from build123d import *

# Parameters (mm, degrees)
SKETCH1_R           = 250
SKETCH1_R_2         = 162.5
BOSS_EXTRUDE1_DEPTH = 19
CUT_EXTRUDE1_START  = -6
SKETCH2_R           = 250
SKETCH2_R_2         = 236
CUT_EXTRUDE1_DEPTH  = 6
SKETCH3_R           = 5
CUT_EXTRUDE2_DEPTH  = 355.063553617


with BuildPart() as part:
    # Sketch1 → Boss-Extrude1 (new body)
    with BuildSketch(Plane(origin=(0, 0, 0), x_dir=(1, 0, 0), z_dir=(0, 1, 0))):
        with Locations(Location((0, 0, 0), (0, 0, 270))):
            Circle(SKETCH1_R)
        with Locations(Location((0, 0, 0), (0, 0, 270))):
            Circle(SKETCH1_R_2, mode=Mode.SUBTRACT)
    extrude(amount=BOSS_EXTRUDE1_DEPTH)

    # Sketch2 → Cut-Extrude1 (cut)
    with BuildSketch(Plane(origin=(0, 19, 0), x_dir=(1, 0, 0), z_dir=(0, 1, 0)).offset(CUT_EXTRUDE1_START)):
        with Locations(Location((0, 0, 0), (0, 0, 270))):
            Circle(SKETCH2_R)
        with Locations(Location((0, 0, 0), (0, 0, 270))):
            Circle(SKETCH2_R_2, mode=Mode.SUBTRACT)
    extrude(amount=CUT_EXTRUDE1_DEPTH, mode=Mode.SUBTRACT)

    # Sketch3 → Cut-Extrude2 (cut, through all)
    with BuildSketch(Plane(origin=(0, 19, 0), x_dir=(1, 0, 0), z_dir=(0, 1, 0))):
        with Locations(Location((111.25, 192.690652342, 0), (0, 0, 270))):
            Circle(SKETCH3_R)
        with Locations(Location((111.25, -192.690652342, 0), (0, 0, 90))):
            Circle(SKETCH3_R)
        with Locations(Location((-111.25, -192.690652342, 0), (0, 0, 270))):
            Circle(SKETCH3_R)
        with Locations(Location((222.5, 0, 0), (0, 0, 270))):
            Circle(SKETCH3_R)
        with Locations(Location((-111.25, 192.690652342, 0), (0, 0, 90))):
            Circle(SKETCH3_R)
        with Locations(Location((-222.5, 0, 0), (0, 0, 90))):
            Circle(SKETCH3_R)
    extrude(amount=-CUT_EXTRUDE2_DEPTH, mode=Mode.SUBTRACT)


solid = part.part
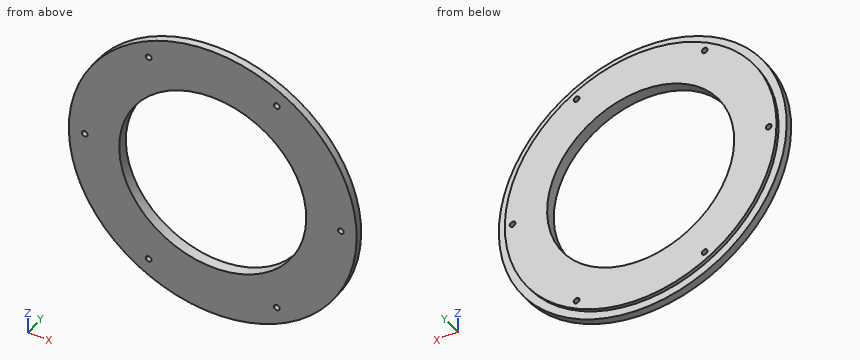
Check sheet for the modelled part. Datum: model origin and axes. Units: mm. Give positions to 0.01 mm unless a question says otherwise; leave off trailing zeros. Loops run counter-clockwise (first coordinate to the right, second up) from the corner with the lowest first, then second, coordinate; pieces in that order, holes last. Notation, with made-up numbers: M -6.75,40 L 5.25,40 A33 ccw 5.25,73 Z; hole C 27.5,22 d6. An arc over 180 degrees is marked long. Answer as a JSON object with one key per item and string values. Group by question number.
Q1. Go/stop test with flat-tipped pins: P1, Ø8, axis at x = -61, y = 13.5, coming from the -Z side; P2, Ø8, axis at y = 10.5, z = -36.5, coming from the -X side; P3, Ø8, axis at y = 3.5, z = 137.5, coming from the +X side; P4, Ø9, axis at x = 111.25, z = -192.69, coming from the +Y side. Record where each tip stops, or that it passes through.
Q2. Material ranges on line 1 along X through (y, z) = (10.25, 0); line 2 along X through (y, z) = (16.25, -189); line 3 along Z through (x, y) = (119, 8.5), recorded low to high. Write a range as [from, to].
Q3. Cross-section at B-B on x = -96.5. Record the cut outline in (y, z).
Q4. Cross-section at A-A on y = 3.5. Record the cut outline in (x, z), then the cut area to 3 significant figures.
Q5. Cross-section at D-D on z = 205.5. Record the cut outline in (x, y), then the cut area to 3 significant figures.
Q6. Cross-section at C-C on z = 44. Record the cut outline in (x, y).
Evaluation:
{
 "1": {"P1": "stops at z = -243.41", "P2": "stops at x = -247.88", "P3": "stops at x = 211.37", "P4": "passes through"},
 "2": {"line 1": "x = [-250, -227.5], [-217.5, -162.5], [162.5, 217.5], [227.5, 250]", "line 2": "x = [-141.33, -114.62], [-107.88, 107.88], [114.62, 141.33]", "line 3": "z = [-219.86, -110.66], [110.66, 219.86]"},
 "3": {"outline": "M 0,-230.62 L 13,-230.62 L 13,-215.37 L 19,-215.37 L 19,-130.74 L 0,-130.74 Z; M 0,130.74 L 19,130.74 L 19,215.37 L 13,215.37 L 13,230.62 L 0,230.62 Z"},
 "4": {"outline": "C 0,0 d500; hole C -222.5,0 d10; hole C 0,0 d325; hole C -111.25,-192.69 d10; hole C -111.25,192.69 d10; hole C 111.25,-192.69 d10; hole C 111.25,192.69 d10; hole C 222.5,0 d10", "area": "113,000 mm2"},
 "5": {"outline": "M -142.37,0 L 142.37,0 L 142.37,13 L 116.04,13 L 116.04,19 L -116.04,19 L -116.04,13 L -142.37,13 Z", "area": "5,090 mm2"},
 "6": {"outline": "M -246.1,0 L -156.43,0 L -156.43,19 L -231.86,19 L -231.86,13 L -246.1,13 Z; M 156.43,0 L 246.1,0 L 246.1,13 L 231.86,13 L 231.86,19 L 156.43,19 Z"}
}
